from build123d import *

# Parameters (mm, degrees)
SKETCH_1_R      = 2.5
EXTRUDE_1_DEPTH = 4
FILLET_1_R      = 2


with BuildPart() as part:
    # ｽｹｯﾁ1 → ﾎﾞｽ - 押し出し1 (new body)
    with BuildSketch(Plane.XY):
        Polygon((0, 0), (0, -9.5), (4.107330666, -9.5), (4.107330666, -15.441500508), (15.922353162, -11.607425741), (15.922353162, 0.037444009), (4, 4.930710615), (4, 0), align=None)
        with Locations((9.4, -4.4)):
            Circle(SKETCH_1_R, mode=Mode.SUBTRACT)
    extrude(amount=EXTRUDE_1_DEPTH)

    # ﾌｨﾚｯﾄ1
    fillet_1_edges = [part.edges().sort_by_distance(p)[0] for p in [
        (15.922353162, 0.037444009, 2),
        (15.922353162, -11.607425741, 2),
    ]]
    fillet(fillet_1_edges, radius=FILLET_1_R)


solid = part.part
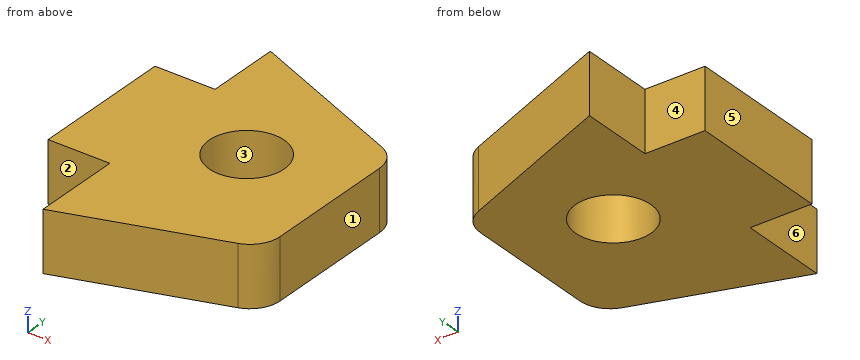
The listing builds one solid part. Answer for the finished solid, in the listing's coordinates (mm). Face numbers are marked on the shaded views. A direction names the side the tool comes from. Coordinates: 2 decimals unless noted, no trailing zeros. Order: outer loops, then holes, each group sorted by start corner. A loop starts at its lowest first (then second) coordinate and runs counter-clockwise, first axis right, second up. Notation, with made-up numbers: M 1.5,19.5 L 25.5,19.5 A17 ccw 25.5,31.5 Z; hole C 58.25,23.5 d1. An arc over 180 degrees is marked long. Use CSV: the item, a comma, the result in double quotes.
Q1. Determine the mould class of the marked faces 1, 2 and 3 for opening direction X: pulls with the +X half, pulls with the -X half, needs draft (parallel to the pull), parting line crosses it, or undercut.
Here are the results:
face 1,"pulls with the +X half"
face 2,"needs draft"
face 3,"undercut"
Q2. Straight lines are drawn through the part: L1, parallel to Y at x = 9.4, z = 2.45; L2, parallel to X at y = -6.25, z = 1.7; L3, parallel to Y at x = 9.75, z = 2.7. For each, find the intervals that lie inside material, in ascending order.
Here are the results:
L1,"-13.72 to -6.9, -1.9 to 2.71"
L2,"0 to 7.72, 11.08 to 15.92"
L3,"-13.61 to -6.88, -1.92 to 2.57"
Q3. A tool of negligible diameter and unlimited length cuts with its end or side. For the marked faces 4, 5 and 6, from which of +Z, -Z, +X, -X, +Y, -Y can it reach the whole face along a straight path? Write none if from no direction.
Here are the results:
face 4,"+Z, -Z, -X, +Y"
face 5,"+Z, -Z, -X, +Y, -Y"
face 6,"+Z, -Z, -X, -Y"
Q4. Section B-B (z = 3.2) is taken. Determine the outline of the cut face in (x, y).
Here are the results:
outline,"M 0,-9.5 L 4.11,-9.5 L 4.11,-15.44 L 14.54,-12.06 A2 ccw 15.92,-10.15 L 15.92,-1.3 A2 ccw 14.68,0.55 L 4,4.93 L 4,0 L 0,0 Z; hole C 9.4,-4.4 d5"
Q5. Section C-C (x = 9.4) is taken. Determine the outline of the cut face in (y, z), then the cut area to 3 significant figures.
Here are the results:
outline,"M -13.72,0 L -6.9,0 L -6.9,4 L -13.72,4 Z; M -1.9,0 L 2.71,0 L 2.71,4 L -1.9,4 Z"
area,"45.8 mm2"
Q6. Given pin 1 Ø2 at (x, y) = (2, 2.5) entering from -Z; pin 2 Ø1.5 at (y, z) = (2.5, 3) entering from +X; pin 3 Ø2 at (x, z) = (13, 0.5) entering from -Y, each flat-ended and moving along its own axis, determine where each tip first touches the part or whether it passes through.
Here are the results:
pin 1,"through"
pin 2,"x = 11.75"
pin 3,"y = -12.88"
Q7. Section A-A (y = -4.4) is taken. Determine the outline of the cut face in (x, z).
Here are the results:
outline,"M 0,0 L 6.9,0 L 6.9,4 L 0,4 Z; M 11.9,0 L 15.92,0 L 15.92,4 L 11.9,4 Z"
Q8. Section D-D (x = 3.75) is taken. Determine the outline of the cut face in (y, z), then the cut area to 3 significant figures.
Here are the results:
outline,"M -9.5,0 L 0,0 L 0,4 L -9.5,4 Z"
area,"38.0 mm2"
